Job drawing, mm, ordinate dimensions from the low corner. One solid piece. A direction names the side the tool comes from. Coordinates: 2 decimals unless noted, no trailing zeros. Order: outer loops, then holes, each group sorted by start corner. A loop starts at its lowest first (then second) coordinate and runs counter-clockwise, first axis right, second up. Notation, with made-up numbers: (56.25, -22.75) -> (99.25, -22.75) arc R14 cw to (99.25, -7.75) -> close; hole circle Ø2 at (63, 83). An arc over 180 degrees is marked (long way). Use CSV: the item, a comma, the result in double quotes. Start each with the question number.
(1) Cut at C-C on y = 2.25. Write the cut outline in (x, z).
(2) Cut at A-A on z = 30. Write the cut outline in (x, y).
(3) Tool access for the marked faces 5 and 6: list every direction of +Z, -Z, +X, -X, +Y, -Y with a clear straight run to the whole face (end or side of a thin tool).
(4) Probe L1, parallel to Z at x = 10.5, y = 4; L2, parallel to X at y = 2.25, z = 24.5; L3, parallel to Y at x = 30, z = 24.5. List the from-to ranges inside material, lowest first.
(5) Pin check, flat tips, straight feed: pin 1 Ø5 at (x, z) = (27.5, 30) entering from -Y; pin 2 Ø3.5 at (x, z) = (28.5, 24) entering from +Y; pin 3 Ø5 at (x, z) = (29.5, 30) entering from +Y. Stop position of each tip, or through.
(6) Cut at B-B on x = 37. Write the cut outline in (y, z).
(7) Pull direction X, two halves, no side cores. Call the marked faces 1, 2, 3 and 4: pulls with the +X half, pulls with the -X half, needs draft (parallel to the pull), parting line crosses it, or undercut.
(8) Cut at D-D on z = 18. Write the cut outline in (x, y), plus the area to 3 significant figures.
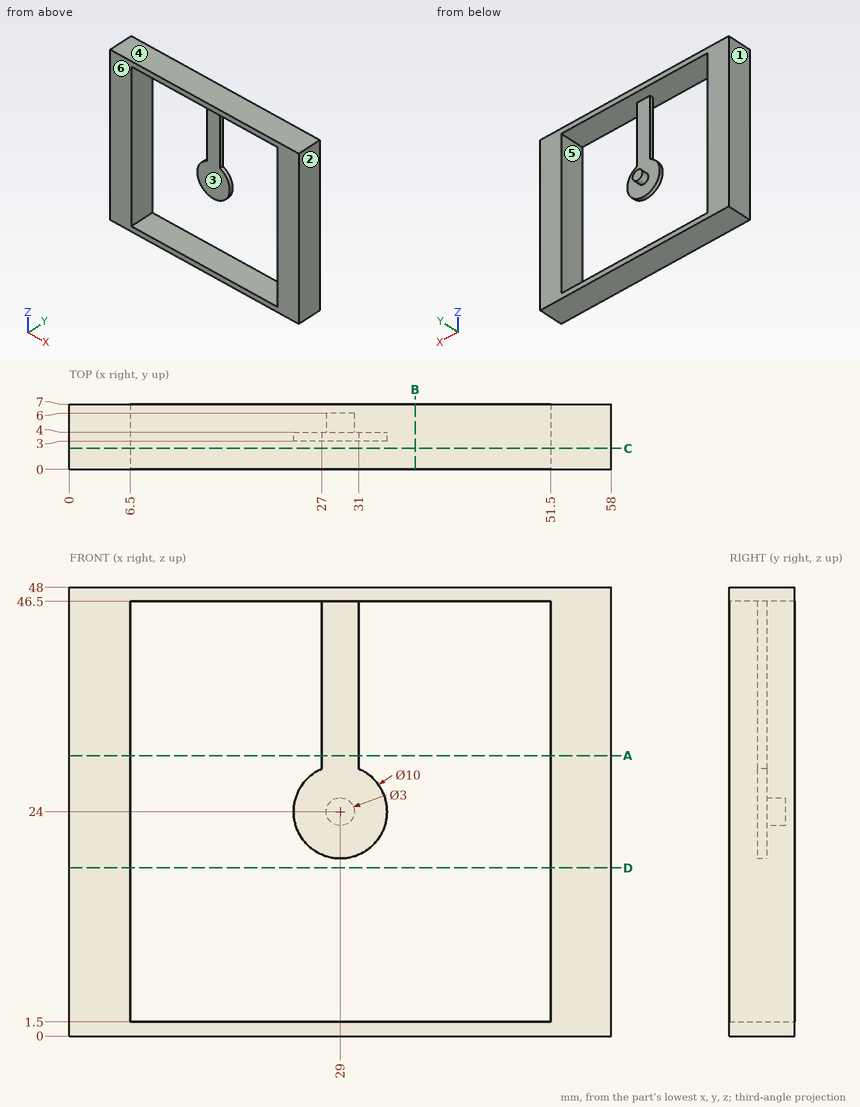
Outcome:
1,outline,"(0, 0) -> (58, 0) -> (58, 48) -> (0, 48) -> close; hole (6.5, 1.5) -> (51.5, 1.5) -> (51.5, 46.5) -> (6.5, 46.5) -> close"
2,outline,"(0, 0) -> (6.5, 0) -> (6.5, 7) -> (0, 7) -> close; (27, 3) -> (31, 3) -> (31, 4) -> (27, 4) -> close; (51.5, 0) -> (58, 0) -> (58, 7) -> (51.5, 7) -> close"
3,face 5,"+Y, -Y"
3,face 6,"+Z, -Z, +X, -X, -Y"
4,L1,"0 to 1.5, 46.5 to 48"
4,L2,"0 to 6.5, 51.5 to 58"
4,L3,"3 to 6"
5,pin 1,"y = 3"
5,pin 2,"y = 6"
5,pin 3,"y = 4"
6,outline,"(0, 0) -> (7, 0) -> (7, 1.5) -> (0, 1.5) -> close; (0, 46.5) -> (7, 46.5) -> (7, 48) -> (0, 48) -> close"
7,face 1,"pulls with the -X half"
7,face 2,"pulls with the +X half"
7,face 3,"undercut"
7,face 4,"needs draft"
8,outline,"(0, 0) -> (6.5, 0) -> (6.5, 7) -> (0, 7) -> close; (51.5, 0) -> (58, 0) -> (58, 7) -> (51.5, 7) -> close"
8,area,"91.0 mm2"
